Work out the finished part from the listing and answer in its coordinate system (mm). Coordinates: 2 decimals unless noted, no trailing zeros. Order: outer loops, then holes, each group sorted by start corner. A loop starts at its lowest first (then second) coordinate and runs counter-clockwise, first axis right, second up. Notation, with made-up numbers: M -1.5,-32 L 24.5,-32 A20 cw 24.5,-18 Z; hole C 50,68.5 d2. An arc over 180 degrees is marked long. Answer in a Markdown table with one row per item. Add a question column.
Item 1: Consider line 1 (Z direction, x = 4.75, y = 49.5); line 2 (Y direction, x = 1.5, z = -26.5) (3 decimals); line 3 (Y direction, x = 2.75, z = 336.55). Determine where each line is inside the solid, lowest interval first. Write a range as from..to.
Item 2: The part is cut by section C-C (y = 83). Write down the section's boundary in (x, z), then the cut area to 3 significant figures.
Item 3: The part is cut by section B-B (y = 160.5). Write down the section's boundary in (x, z).
Item 4: Flat-ended cylindrical pins translate along their axes: pin 1 Ø4 at (y, z) = (19.05, -171.45) entering from -X; pin 2 Ø1.9 at (x, z) = (1.5, 25) entering from -Y; pin 3 Ø3 at (x, z) = (2, -141) entering from +Y. Find the tip coordinate at first contact, or state that the pin passes through.
Item 5: The part is cut by section A-A (x = 1.5). State how many separate pieces and enclosed holes the cut face has, then the cut area to 3 significant figures.
from build123d import *

# Parameters (mm, degrees)
BOSS_EXTRUDE1_DEPTH     = 6.35
SKETCH2_W               = 203.2
SKETCH2_H               = 50.8
CUT_EXTRUDE1_DEPTH      = 696.81774778
F_1_4_CLEARANCE_HOLE1_D = 6.7564
FILLET1_R               = 3.302


with BuildPart() as part:
    # Sketch1 → Boss-Extrude1 (new body)
    with BuildSketch(Plane(origin=(0, 0, 0), x_dir=(0, 0, -1), z_dir=(1, 0, 0))):
        Polygon((89.265604664, 219.075), (-89.265604664, 219.075), (-660.4, 66.04), (-660.4, 0), (660.4, 0), (660.4, 66.04), align=None)
    extrude(amount=BOSS_EXTRUDE1_DEPTH)

    # Sketch2 → Cut-Extrude1 (cut, through all)
    with BuildSketch(Plane(origin=(6.35, 0, 0), x_dir=(0, 0, -1), z_dir=(1, 0, 0))):
        with Locations((0, 25.4)):
            Rectangle(SKETCH2_W, SKETCH2_H)
    extrude(amount=-CUT_EXTRUDE1_DEPTH, mode=Mode.SUBTRACT)

    # 1/4 Clearance Hole1 (through all)
    with Locations(Plane.ZY):
        with Locations((-336.55, 19.05), (-120.65, 19.05), (120.65, 19.05), (336.55, 19.05), (0, 114.3), (-171.45, 19.05), (171.45, 19.05)):
            Hole(F_1_4_CLEARANCE_HOLE1_D / 2)

    # Fillet1
    fillet1_edges = [part.edges().sort_by_distance(p)[0] for p in [
        (3.175, 66.04, 660.4),
        (3.175, 219.075, 89.265604664),
        (3.175, 219.075, -89.265604664),
        (3.175, 66.04, -660.4),
        (3.175, 0, -660.4),
        (3.175, 0, 660.4),
        (3.175, 0, -101.6),
        (3.175, 0, 101.6),
        (3.175, 50.8, 101.6),
        (3.175, 50.8, -101.6),
    ]]
    fillet(fillet1_edges, radius=FILLET1_R)


solid = part.part
Reply:
| question | item | result |
|---|---|---|
| 1 | line 1 | z = -660.4..-100.92, 100.92..660.4 |
| 1 | line 2 | y = 50.8..219.075 |
| 1 | line 3 | y = 0..15.67, 22.43..152.82 |
| 2 | outline | M 0,-597.1 L 6.35,-597.1 L 6.35,597.1 L 0,597.1 Z |
| 2 | area | 7,580 mm2 |
| 3 | outline | M 0,-307.87 L 6.35,-307.87 L 6.35,307.87 L 0,307.87 Z |
| 4 | pin 1 | passes through |
| 4 | pin 2 | stops at y = 50.8 |
| 4 | pin 3 | stops at y = 205.61 |
| 5 | separate pieces | 1 |
| 5 | enclosed holes | 7 |
| 5 | area | 191,000 mm2 |
